Geometry: final body of the model. Coordinates: model frame, mm. Face numbers are marked on the shaded views. A direction names the side the tool comes from. Coordinates: 2 decimals unless noted, no trailing zeros. Order: outer loops, then holes, each group sorted by start corner. A loop starts at its lowest first (then second) coordinate and runs counter-clockwise, first axis right, second up. Notation, with made-up numbers: (-16, -15.75) - (40, -15.75) arc R15 ccw to (40, 2.25) - close; hole circle Ø9 at (-36, -22). An arc over 180 degrees is marked (long way). Use a Markdown table: item, result. Add a question column.
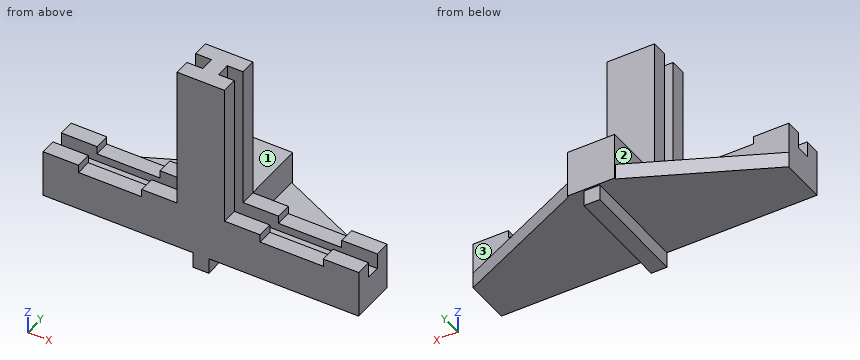
```python
from build123d import *

# Parameters (mm, degrees)
F0_W      = 2
F0_H      = 2
F1_DEPTH  = 24
F0_W_2    = 17
F2_DEPTH  = 6
F0_H_2    = 1.8
F3_DEPTH  = 4
F4_W      = 6
F4_H      = 6
F5_DEPTH  = 14
F6_DEPTH  = 2
F7_DEPTH  = 2
F8_DEPTH  = 2
F9_W      = 8
F9_H      = 1
F10_DEPTH = 6
F11_DEPTH = 2
F12_DEPTH = 2


with BuildPart() as f1:
    # F0 (on Top) → F1 (new body)
    with BuildSketch(Plane.XY):
        with Locations((18, -1)):
            Rectangle(F0_W, F0_H)
        Polygon((20, 0), (19, 0), (19, -2), (20, -2), (21, -2), (21, 0), align=None)
        with Locations((22, -1)):
            Rectangle(F0_W, F0_H)
        Polygon((20, -2), (19, -2), (19, -3.8), (20, -3.8), (21, -3.8), (21, -2), align=None)
        with Locations((18, -4.8)):
            Rectangle(F0_W, F0_H)
        Polygon((20, -3.8), (19, -3.8), (19, -5.8), (20, -5.8), (21, -5.8), (21, -3.8), align=None)
        with Locations((22, -4.8)):
            Rectangle(F0_W, F0_H)
    extrude(amount=F1_DEPTH)

    # F0 (on Top) → F2 (join)
    with BuildSketch(Plane.XY):
        with Locations((8.5, -1)):
            Rectangle(F0_W_2, F0_H)
        with Locations((8.5, -4.8)):
            Rectangle(F0_W_2, F0_H)
        with Locations((31.5, -1)):
            Rectangle(F0_W_2, F0_H)
        with Locations((31.5, -4.8)):
            Rectangle(F0_W_2, F0_H)
    extrude(amount=F2_DEPTH)

    # F0 (on Top) → F3 (join)
    with BuildSketch(Plane.XY):
        with Locations((8.5, -2.9)):
            Rectangle(F0_W_2, F0_H_2)
        with Locations((18, -2.9)):
            Rectangle(F0_W, F0_H_2)
        with Locations((22, -2.9)):
            Rectangle(F0_W, F0_H_2)
        with Locations((31.5, -2.9)):
            Rectangle(F0_W_2, F0_H_2)
    extrude(amount=F3_DEPTH)

    # F4 (on face) → F5 (join)
    with BuildSketch(Plane.XZ.offset(5.8)):
        with Locations((20, 3)):
            Rectangle(F4_W, F4_H)
    extrude(amount=-F5_DEPTH)

    # F0 (on Top) → F6 (join)
    with BuildSketch(Plane.XY):
        Polygon((20, -3.8), (19, -3.8), (19, -5.8), (20, -5.8), (21, -5.8), (21, -3.8), align=None)
        Polygon((20, -2), (19, -2), (19, -3.8), (20, -3.8), (21, -3.8), (21, -2), align=None)
        Polygon((20, 0), (19, 0), (19, -2), (20, -2), (21, -2), (21, 0), align=None)
        Polygon((19, 8), (19, 0), (20, 0), (21, 0), (21, 8), align=None)
    extrude(amount=-F6_DEPTH)

    # F7 (cut): a face of the model
    f7_faces = [f1.faces().sort_by_distance(p)[0] for p in [
        (17, -2.9, 5),
    ]]
    extrude(f7_faces, amount=-F7_DEPTH, mode=Mode.SUBTRACT)

    # F8 (cut): a face of the model
    f8_faces = [f1.faces().sort_by_distance(p)[0] for p in [
        (23, -2.9, 5),
    ]]
    extrude(f8_faces, amount=-F8_DEPTH, mode=Mode.SUBTRACT)

    # F9 (on face) → F10 (cut)
    with BuildSketch(Plane.XZ.offset(5.8)):
        with Locations((8.5, 5.5)):
            Rectangle(F9_W, F9_H)
        with Locations((8.5, 6.5)):
            Rectangle(F9_W, F9_H)
        with Locations((31.5, 6.5)):
            Rectangle(F9_W, F9_H)
        with Locations((31.5, 5.5)):
            Rectangle(F9_W, F9_H)
    extrude(amount=-F10_DEPTH, mode=Mode.SUBTRACT)

    # F0 (on Top) → F11 (join)
    with BuildSketch(Plane.XY):
        Polygon((17, 8), (0, 0), (17, 0), align=None)
    extrude(amount=F11_DEPTH)

    # F0 (on Top) → F12 (join)
    with BuildSketch(Plane.XY):
        Polygon((40, 0), (23, 8), (23, 0), align=None)
    extrude(amount=F12_DEPTH)


solid = f1.part
```
1) Section A-A (y = 6). Return loops of the section in (x, z), then the cut area to 3 significant figures.
2) Section B-B (z = 1). Return loops of the section in (x, y).
3) Pin query (flat end, axial travel): pin 1 (0.6 mm diameter, centred on x = 26.5, y = -4.5, fed in from +Z); pin 2 (6 mm diameter, centred on x = 34, y = -2.5, fed in from -Z); pin 3 (0.6 mm diameter, centred on x = 33.5, y = -1, fed in from +Z). Return the tip coordinate at first contact, or that it passes through.
4) Section C-C (x = 25). Return loops of the section in (y, z), then the cut area to 3 significant figures.
5) Ray query, line 1 along Y through (x, z) = (3, 4.5); line 2 along X through (y, z) = (-5, 21.75); line 3 along Z through (x, y) = (15, 4). Return the intervals inside material, ascending.
6) Set-up query: the marked faces 1, 2 and 3. Return all of +Z, -Z, +X, -X, +Y, -Y with unobstructed straight access to the full face (end or side cutting, diameter ignored); none if empty.
7) Section D-D (z = 12.75). Return loops of the section in (x, y), then the cut area to 3 significant figures.
Values follow:
| question | item | result |
|---|---|---|
| 1 | outline | (12.75, 0) - (19, 0) - (19, -2) - (21, -2) - (21, 0) - (27.25, 0) - (27.25, 2) - (23, 2) - (23, 6) - (17, 6) - (17, 2) - (12.75, 2) - close |
| 1 | area | 57.0 mm² |
| 2 | outline | (0, -5.8) - (40, -5.8) - (40, 0) - (23, 8) - (23, 8.2) - (17, 8.2) - (17, 8) - (0, 0) - close |
| 3 | pin 1 | stops at z = 6 |
| 3 | pin 2 | stops at z = 0 |
| 3 | pin 3 | stops at z = 5 |
| 4 | outline | (-5.8, 0) - (7.06, 0) - (7.06, 2) - (0, 2) - (0, 6) - (-2, 6) - (-2, 4) - (-3.8, 4) - (-3.8, 6) - (-5.8, 6) - close |
| 4 | area | 45.3 mm² |
| 5 | line 1 | y = -5.8 to -3.8, -2 to 0 |
| 5 | line 2 | x = 17 to 23 |
| 5 | line 3 | z = 0 to 2 |
| 6 | face 1 | +Z, +X, -X, +Y |
| 6 | face 2 | +Z, -X, +Y |
| 6 | face 3 | +Z, +X, +Y |
| 7 | outline | (17, -5.8) - (23, -5.8) - (23, -3.8) - (21, -3.8) - (21, -2) - (23, -2) - (23, 0) - (17, 0) - (17, -2) - (19, -2) - (19, -3.8) - (17, -3.8) - close |
| 7 | area | 27.6 mm² |
